Autodesk Inventor part; units mm, degrees
ref_plane "YZ Plane" through (0, 0, 0) normal (1, 0, 0) x (0, 1, 0)
ref_plane "XZ Plane" through (0, 0, 0) normal (0, 1, 0) x (-1, 0, 0)
ref_plane "XY Plane" through (0, 0, 0) normal (0, 0, 1) x (1, 0, 0)
sketch "Skizze1" plane through (0, 0, 0) normal (0, 1, 0) x (-1, 0, 0)
  line L0 (40.25, -10.25) -> (-40.25, -10.25)
  line L1 (-40.25, -10.25) -> (-40.25, 10.25)
  line L2 (-40.25, 10.25) -> (40.25, 10.25)
  line L3 (40.25, 10.25) -> (40.25, -10.25)
  line L4 (40.25, -10.25) -> (-40.25, 10.25) construction
  line L5 (-40.25, -10.25) -> (40.25, 10.25) construction
  line L6 (42.65, -12.65) -> (-42.65, -12.65)
  line L7 (-42.65, -12.65) -> (-42.65, 12.65)
  line L8 (-42.65, 12.65) -> (42.65, 12.65)
  line L9 (42.65, 12.65) -> (42.65, -12.65)
  line L10 (37.85, -7.85) -> (-37.85, -7.85)
  line L11 (-37.85, -7.85) -> (-37.85, 7.85)
  line L12 (-37.85, 7.85) -> (37.85, 7.85)
  line L13 (37.85, 7.85) -> (37.85, -7.85)
  line L14 (52.65, -12.65) -> (42.65, -12.65)
  line L15 (42.65, 12.65) -> (52.65, 12.65)
  circle A0 centre (52.65, 0) radius 2
  line L16 (-42.65, -12.65) -> (-52.65, -12.65)
  line L17 (-42.65, 12.65) -> (-52.65, 12.65)
  circle A1 centre (-52.65, 0) radius 2
  arc A2 (62.65, 2.65) -> (52.65, 12.65) centre (52.65, 2.65) ccw
  arc A3 (52.65, -12.65) -> (62.65, -2.65) centre (52.65, -2.65) ccw
  line L18 (62.65, 2.65) -> (62.65, -2.65)
  arc A4 (-52.65, 12.65) -> (-62.65, 2.65) centre (-52.65, 2.65) ccw
  arc A5 (-62.65, -2.65) -> (-52.65, -12.65) centre (-52.65, -2.65) ccw
  line L19 (-62.65, 2.65) -> (-62.65, -2.65)
  point P0 (0, 0)
  point P1 (62.65, 0)
  point P2 (-62.65, 0)
  dimension "d0" = 80.5
  dimension "d1" = 20.5
  dimension "d2" = 2.4
  dimension "d3" = 2.4
  dimension "d4" = 4
  dimension "d7" = 4
  dimension "d25" = 20
  dimension "d26" = 10
  dimension "d27" = 10
  dimension "d28" = 20
  dimension "d29" = 10
  dimension "d30" = 10
extrude "Extrusion1" add sketch "Skizze1" against normal blind 2 contours L0 L1 L2 L3 | L6 L7 L8 L9 | L9 L15 A2 L18 A3 L14 | L16 A5 L19 A4 L17 L7 | L10 L11 L12 L13
extrude "Extrusion2" add sketch "Skizze1" along normal blind 5 contours L6 L7 L8 L9 | L9 L15 A2 L18 A3 L14 | L16 A5 L19 A4 L17 L7
extrude "Extrusion3" add sketch "Skizze1" along normal blind 2 contours L0 L1 L2 L3
sketch "Skizze2" plane through (0, 0, 0) normal (0, 0, 1) x (1, 0, 0)
  line L0 (37.85, 0) -> (37.85, 2)
  line L1 (37.85, 2) -> (40.25, 2)
  line L2 (40.25, 2) -> (40.25, 5)
  line L3 (40.25, 5) -> (50.65, 5)
  line L4 (50.65, 5) -> (50.65, -2)
  line L5 (50.65, -2) -> (-50.65, -2)
  line L6 (-50.65, -2) -> (-50.65, 5)
  line L7 (-50.65, 5) -> (-40.25, 5)
  line L8 (-40.25, 5) -> (-40.25, 2)
  line L9 (-40.25, 2) -> (-37.85, 2)
  line L10 (-37.85, 2) -> (-37.85, 0)
  line L11 (-37.85, 0) -> (37.85, 0)
  line L12 (-62.65, 5) -> (-54.65, 5)
  line L13 (-54.65, 5) -> (-54.65, -2)
  line L14 (-54.65, -2) -> (-62.65, -2)
  line L15 (54.65, 5) -> (62.65, 5)
  line L16 (62.65, -2) -> (54.65, -2)
  line L17 (54.65, -2) -> (54.65, 5)
  arc A0 (-40.25, 3.5) -> (-40.25, 5) centre (-40.25, 4.25) ccw
  arc A1 (40.25, 5) -> (40.25, 3.5) centre (40.25, 4.25) ccw
  line L18 (-40.25, 5) -> (-40.25, 3.5)
  line L19 (40.25, 5) -> (40.25, 3.5)
  line L20 (-62.65, -2) -> (-62.65, 5)
  line L21 (62.65, 5) -> (62.65, -2)
  line L22 (-40.25, 3.5) -> (40.25, 3.5)
  line L23 (40.25, 5) -> (-40.25, 5)
  line L24 (-39.5, 4.25) -> (-39.5, 3.5)
  line L25 (39.5, 4.25) -> (39.5, 3.5)
  point P0 (0, 0)
  dimension "d14" = 1.5
  dimension "d15" = 1.5
extrude "Extrusion4" add sketch "Skizze2" along normal mid plane 20.5 contours A1 L2 | L8 A0
sketch "Skizze3" plane through (0, 5, 0) normal (0, 1, 0) x (1, 0, 0)
  circle A0 centre (-52.65, 0) radius 2
  circle A1 centre (52.65, 0) radius 2
  point P0 (0, 0)
hole "Bohrung1" at (-52.65, 5, 0) at (52.65, 5, 0) direction (0, -1, 0) diameter 4.5 depth 6 countersink diameter 9.4 countersink angle 90
extrude "Extrusion5" cut sketch "Skizze2" along normal through all both and the other way through all contours A1 L25 L22 L24 A0 L23
equation "\"d7\" = d4"
equation "\"d28\" = d25"
equation "\"d29\" = d27"
equation "\"d30\" = d26"
equation "\"d15\" = d14"
properties part number "PCB_Holder_A"
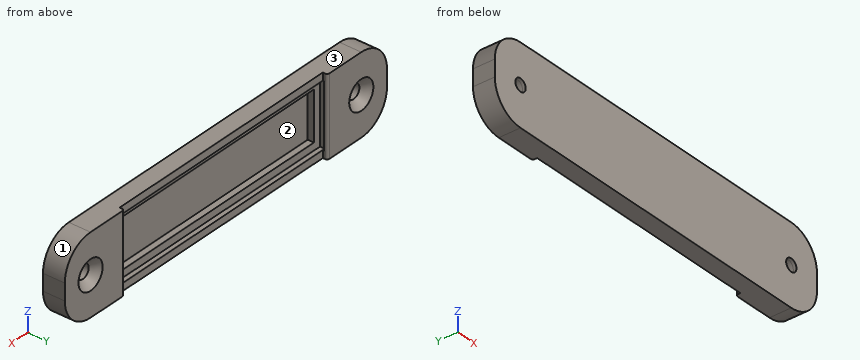
The listing builds one solid part. Answer for the finished solid, in the listing's coordinates (mm). Face numbers are marked on the shaded views. Coordinates: 2 decimals unless noted, no trailing zeros. Write each loop counter-clockwise with the first axis right and the second up, starting at its lowest first coordinate (ties: lowest second). Pieces come first, ordered by that corner, then holes. Notation, with made-up numbers: M -31.5,14.25 L -25.5,14.25 A24 cw -25.5,44.25 Z; hole C 43.25,-35.5 d6. An arc over 180 degrees is marked long. Write each question's results on one line, items separated by ' | '.
Item 1: Consider probe 1 along X at (y, z) = (0.6, 0); probe 2 along X at (y, z) = (-1.2, 0); probe 3 along X at (y, z) = (4.75, -0.5). Determine where each line is inside the solid, lowest interval first. Write a range as [from, to].
Answer below:
probe 1: [-62.65, -54.9], [-50.4, -37.85], [37.85, 50.4], [54.9, 62.65] | probe 2: [-62.65, -54.65], [-50.65, 50.65], [54.65, 62.65] | probe 3: [-62.65, -57.07], [-48.23, -39.69], [39.69, 48.23], [57.07, 62.65]
Item 2: For a pull along X with two mould halves and no side action, classify the marked faces 1, 2 and 3 as released by +X, released by -X, zero draft, split by the parting line, or undercut.
Answer below:
face 1: released by +X | face 2: undercut | face 3: zero draft
Item 3: Given P1, Ø5, axis at x = 14.5, z = -1, coming from the +Y side; P2, Ø5, axis at x = -29, z = 6, coming from the +Y side; P3, Ø0.8, axis at y = 4, z = -11.5, coming from the +X side, each flat-ended and moving along its own axis, determine where each tip first touches the part or whether it passes through.
Answer below:
P1: y = 0 | P2: y = 2 | P3: x = 58
Item 4: The part is cut by section A-A on z = 0. State how many separate pieces and enclosed holes the cut face has, and give its area (3 significant figures).
Answer below:
separate pieces: 3 | enclosed holes: 0 | area: 412 mm2
Item 5: The part is cut by section B-B on x = -8.5. Determine the outline of the cut face in (y, z).
Answer below:
outline: M -2,-12.65 L 3.5,-12.65 L 3.5,-10.25 L 2,-10.25 L 2,-7.85 L 0,-7.85 L 0,7.85 L 2,7.85 L 2,10.25 L 3.5,10.25 L 3.5,12.65 L -2,12.65 Z
